Here's how the part is built. I have some questions about the finished solid (model axes, mm). A direction names the side the tool comes from. Round coordinates to 2 decimals unless told otherwise and drop trailing zeros. Loops run counter-clockwise (first coordinate to the right, second up) from the corner with the lowest first, then second, coordinate; pieces in that order, holes last. Notation, with made-up numbers: M -7.75,38.5 L 48.25,38.5 A16 cw 48.25,64.5 Z; hole C -36,61 d2. An arc over 180 degrees is marked long. Answer as a JSON object with one key per item and string values.
Autodesk Inventor part; units mm, degrees
ref_plane "YZ Plane" through (0, 0, 0) normal (1, 0, 0) x (0, 1, 0)
ref_plane "XZ Plane" through (0, 0, 0) normal (0, 1, 0) x (-1, 0, 0)
ref_plane "XY Plane" through (0, 0, 0) normal (0, 0, 1) x (1, 0, 0)
sketch "Sketch1" plane through (0, 0, 0) normal (0, 0, 1) x (1, 0, 0)
  line L0 (-3, 3) -> (3, -3) construction
  line L1 (3, 3) -> (-3, -3) construction
  line L2 (0, 1) -> (3, 1)
  line L3 (3, 1) -> (3, -1)
  line L4 (3, -1) -> (0, -1)
  line L5 (0, -1) -> (0, 1)
  line L6 (0, 1) -> (3, -1) construction
  line L7 (3, 1) -> (0, -1) construction
  line L8 (0, 1) -> (0, 2)
  line L9 (0, 2) -> (1.5, 0)
  line L10 (0, -1) -> (0, -2)
  line L11 (0, -2) -> (1.5, 0)
  point P0 (0, 0)
  point P1 (0, 0)
  point P2 (0.75, 1)
  point P3 (0.75, -1)
  dimension "d0" = 6
  dimension "d1" = 2
  dimension "d2" = 3
  dimension "d3" = 1
extrude "Extrusion1" add sketch "Sketch1" along normal blind 6
sketch "Sketch2" plane through (3, -1, 0) normal (1, 0, 0) x (0, 0, -1)
  point P0 (0, 1)
sketch "Sketch3" plane through (0.75, 1, 0) normal (0, 1, 0) x (1, 0, 0)
  circle A0 centre (5.25, -3) radius 3
  line L0 (2.25, 0) -> (2.25, -6)
  line L1 (2.25, 0) -> (2.25, -6)
  line L2 (2.25, -6) -> (0, -6)
  line L3 (5.25, -6) -> (2.25, -6)
  line L4 (5.25, 0) -> (2.25, 0)
  line L5 (2.25, -6) -> (2.25, 0)
  circle A1 centre (5.25, -3) radius 1
  point P0 (-0.75, 0)
  point P1 (2.25, -3)
  point P2 (2.25, -3)
  dimension "d6" = 6
  dimension "d7" = 2
extrude "Extrusion2" add sketch "Sketch3" against normal up to surface (2 mm away)
properties part number "LinearSlider"
Item 1: I want a section at D-D on z = 4.2. List the corners of the cut face in (x, y) for me.
Solution:
{"outline": "M 0,-2 L 0.75,-1 L 8.75,-1 L 8.75,1 L 0.75,1 L 0,2 Z"}
Item 2: I want a section at B-B on y = -0.4. List the corners of the cut face in (x, z) for me.
Solution:
{"outline": "M 0,0 L 6,0 A3 ccw 6,6 L 0,6 Z; hole C 6,3 d2"}
Item 3: We'd pull the mould along Z, two halves only. Please class faces 4 (the face through (0.37, -1.507, 2.958)), 5 (the face through (5.2, 0, 3.6)), 6 (the face through (3, 0, 0)), 7 (the face through (3, 0, 6)): +Z half, -Z half, draft (parallel to the pull), parting line (faces both ways), or undercut.
Solution:
{"face 4": "draft", "face 5": "undercut", "face 6": "-Z half", "face 7": "+Z half"}
Item 4: For faces 1 (the face through (4.8, 1, 3)), 2 (the face through (4, -1, 3)), 3 (the face through (9, 0, 3)), which set-ups out of +Z, -Z, +X, -X, +Y, -Y let a thin tool reach every point of the face, with its end or its side?
Solution:
{"face 1": "+Z, -Z, +X, +Y", "face 2": "+Z, -Z, +X, -Y", "face 3": "+X, +Y, -Y"}
Item 5: For P1, Ø1.8, axis at x = 4, z = 2, coming from the -Y side; P2, Ø3, axis at x = 6, z = 3, coming from the +Y side, each with a flat end and sliding along its axis, tell me the tip position at first contact or that it passes through.
Solution:
{"P1": "stops at y = -1", "P2": "stops at y = 1"}
Item 6: I want a section at A-A on z = 3. List the corners of the cut face in (x, y) for me.
Solution:
{"outline": "M 0,-2 L 0.75,-1 L 5,-1 L 5,1 L 0.75,1 L 0,2 Z; M 7,-1 L 9,-1 L 9,1 L 7,1 Z"}
Item 7: I want a section at C-C on x = 5.25. List the corners of the cut face in (y, z) for me.
Solution:
{"outline": "M -1,0 L 1,0 L 1,2.34 L -1,2.34 Z; M -1,3.66 L 1,3.66 L 1,6 L -1,6 Z"}
Item 8: If I drill on L1, parallel to X at y = -0.2, z = 3; L2, parallel to Y at x = 2, z = 4.85; L3, parallel to Z at x = 6, y = 0.25, over which ranges is the centre line in solid material (lowest first)? Write a range as from..to.
Solution:
{"L1": "x = 0..5, 7..9", "L2": "y = -1..1", "L3": "z = 0..2, 4..6"}
